```python
from build123d import *

# Parameters (mm, degrees)
SKETCH_1_W          = 135
SKETCH_1_H          = 110
EXTRUDE_1_DEPTH     = 5
SKETCH_2_W          = 20
SKETCH_2_H          = 4.5
EXTRUDE_2_DEPTH     = 20
SKETCH_3_R          = 1.7
CUT_EXTRUDE_1_DEPTH = 130
SKETCH_4_R          = 45.1
SKETCH_4_R_2        = 32.45
CUT_EXTRUDE_2_DEPTH = 2


with BuildPart() as part:
    # 草图1 → 凸台-拉伸1 (new body)
    with BuildSketch(Plane(origin=(0, 0, 0), x_dir=(1, 0, 0), z_dir=(0, 1, 0))):
        Rectangle(SKETCH_1_W, SKETCH_1_H)
    extrude(amount=EXTRUDE_1_DEPTH)

    # 草图2 → 凸台-拉伸2 (add)
    with BuildSketch(Plane(origin=(0, 5, 0), x_dir=(1, 0, 0), z_dir=(0, 1, 0))):
        with Locations((57.5, 52.75)):
            Rectangle(SKETCH_2_W, SKETCH_2_H)
        with Locations((-57.5, 52.75)):
            Rectangle(SKETCH_2_W, SKETCH_2_H)
        with Locations((-57.5, -52.75)):
            Rectangle(SKETCH_2_W, SKETCH_2_H)
        with Locations((57.5, -52.75)):
            Rectangle(SKETCH_2_W, SKETCH_2_H)
    extrude(amount=EXTRUDE_2_DEPTH)

    # 草图3 → 切除-拉伸1 (cut)
    with BuildSketch(Plane(origin=(0, 0, -55), x_dir=(-1, 0, 0), z_dir=(0, 0, -1))):
        with Locations((57.5, 21)):
            Circle(SKETCH_3_R)
        with Locations((51.5, 11)):
            Circle(SKETCH_3_R)
        with Locations((63.5, 11)):
            Circle(SKETCH_3_R)
        with Locations((-51.5, 11)):
            Circle(SKETCH_3_R)
        with Locations((-63.5, 11)):
            Circle(SKETCH_3_R)
        with Locations((-57.5, 21)):
            Circle(SKETCH_3_R)
    extrude(amount=-CUT_EXTRUDE_1_DEPTH, mode=Mode.SUBTRACT)

    # 草图4 → 切除-拉伸2 (cut)
    with BuildSketch(Plane.XZ):
        with Locations(Location((0, 0, 0), (0, 0, 270))):
            Circle(SKETCH_4_R)
        with Locations(Location((0, 0, 0), (0, 0, 270))):
            Circle(SKETCH_4_R_2, mode=Mode.SUBTRACT)
    extrude(amount=-CUT_EXTRUDE_2_DEPTH, mode=Mode.SUBTRACT)


solid = part.part
```
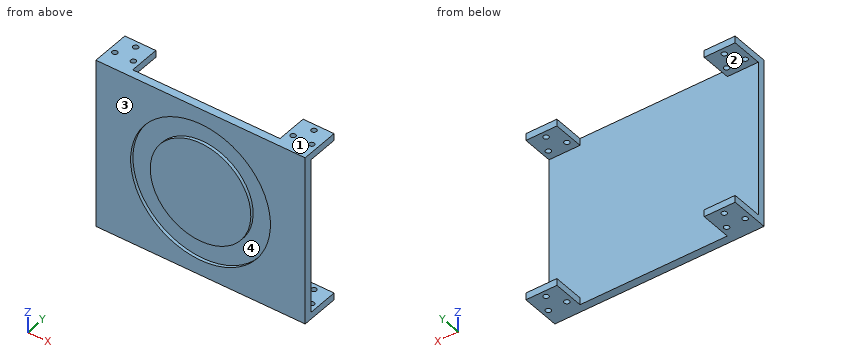
The model under review builds one solid part; all positions refer to its coordinate system, in mm. Face numbers are marked on the shaded views. A direction names the side the tool comes from. Round coordinates to 2 decimals unless told otherwise and drop trailing zeros. Loops run counter-clockwise (first coordinate to the right, second up) from the corner with the lowest first, then second, coordinate; pieces in that order, holes last.
Item 1: Take a section at B-B (y = 21). Give the number of separate pieces and of enclosed holes in the cut face, then the cut area to 3 significant figures.
Determined:
separate pieces: 8
enclosed holes: 0
area: 299 mm2
Item 2: For line 1 (Y direction, x = 63.5, z = -51.6); line 2 (Z direction, x = 59.5, y = 15); line 3 (Y direction, x = 57.5, z = 52.45), list the stretches that pass through material, from the lowest coordinate up.
Determined:
line 1: y = 0 to 9.3, 12.7 to 25
line 2: z = -55 to -50.5, 50.5 to 55
line 3: y = 0 to 19.3, 22.7 to 25
Item 3: Take a section at C-C (z = 0). Write out the cut boundary in (x, y).
Determined:
outline: (-67.5, 0) - (-45.1, 0) - (-45.1, 2) - (-32.45, 2) - (-32.45, 0) - (32.45, 0) - (32.45, 2) - (45.1, 2) - (45.1, 0) - (67.5, 0) - (67.5, 5) - (-67.5, 5) - close
Item 4: Mouldability with a two-part tool opening along X and no side actions: class the marked faces 3 and 4 as released by +X, released by -X, zero draft, split by the parting line, or undercut.
Determined:
face 3: zero draft
face 4: undercut
Item 5: Take a section at D-D (x = 0). Write out the cut boundary in (y, z).
Determined:
outline: (0, -55) - (5, -55) - (5, 55) - (0, 55) - (0, 45.1) - (2, 45.1) - (2, 32.45) - (0, 32.45) - (0, -32.45) - (2, -32.45) - (2, -45.1) - (0, -45.1) - close
Item 6: Take a section at A-A (x = 51.5). Write out the cut boundary in (y, z).
Determined:
outline: (0, -55) - (9.3, -55) - (9.3, -50.5) - (5, -50.5) - (5, 50.5) - (9.3, 50.5) - (9.3, 55) - (0, 55) - close; (12.7, -55) - (25, -55) - (25, -50.5) - (12.7, -50.5) - close; (12.7, 50.5) - (25, 50.5) - (25, 55) - (12.7, 55) - close
Item 7: Clearance check with flat-ended pins moving along their axes: pin 1 Ø4 at (x, y) = (51.5, 11) entering from -Z; pin 2 Ø5 at (x, z) = (20, 31) entering from +Y. State where each tip first meets the part, or that it passes through.
Determined:
pin 1: stops at z = -55
pin 2: stops at y = 5
Item 8: For the marked faces 1 and 2, list the 3-axis set-ups (+Z, -Z, +X, -X, +Y, -Y) from which the entire face can be reached by the end or side of a thin tool; tool diameter is ignored.
Determined:
face 1: +Z, +X, -X, +Y, -Y
face 2: +X, -X, +Y
